Geometry: final body of the model. Coordinates: model frame, mm. Face numbers are marked on the shaded views. A direction names the side the tool comes from. Give positions to 0.01 mm unless a question says otherwise; leave off trailing zeros. Loops run counter-clockwise (first coordinate to the right, second up) from the corner with the lowest first, then second, coordinate; pieces in that order, holes last.
from build123d import *

# Parameters (mm, degrees)
CYLINDER028_R     = 1.25
CYLINDER028_DEPTH = 10
BOX030_W          = 34
BOX030_H          = 2.75
BOX030_DEPTH      = 2
CYLINDER025_W     = 4
CYLINDER025_H     = 26
CYLINDER025_ANGLE = 180


with BuildPart() as b_no002:
    # Cylinder028 → Cylinder028 (new body)
    with BuildSketch(Plane(origin=(11, 29, 4), x_dir=(1, 0, 0), z_dir=(0, 0, 1))):
        Circle(CYLINDER028_R)
    extrude(amount=CYLINDER028_DEPTH)


with BuildPart() as n016:
    # Box030 → Box030 (new body)
    with BuildSketch(Plane(origin=(-3, 25.25, 10), x_dir=(1, 0, 0), z_dir=(0, 0, 1))):
        with Locations((17, 1.375)):
            Rectangle(BOX030_W, BOX030_H)
    extrude(amount=BOX030_DEPTH)


with BuildPart() as obj1:
    # Cylinder025 → Cylinder025 (revolve)
    with BuildSketch(Plane(origin=(11, 28, -14), x_dir=(1, 0, 0), z_dir=(0, -1, 0))):
        with Locations((2, 13)):
            Rectangle(CYLINDER025_W, CYLINDER025_H)
    revolve(axis=Axis((11, 28, -14), (0, 0, 1)), revolution_arc=CYLINDER025_ANGLE)

    # Fusion005: union N016
    add(n016.part)

    # Cut011: cut B_NO002
    add(b_no002.part, mode=Mode.SUBTRACT)


with BuildPart() as obj1_1:
    # Cut011 placement: moved
    add(obj1.part.moved(Location((13, 15, 0))))


solid = obj1_1.part
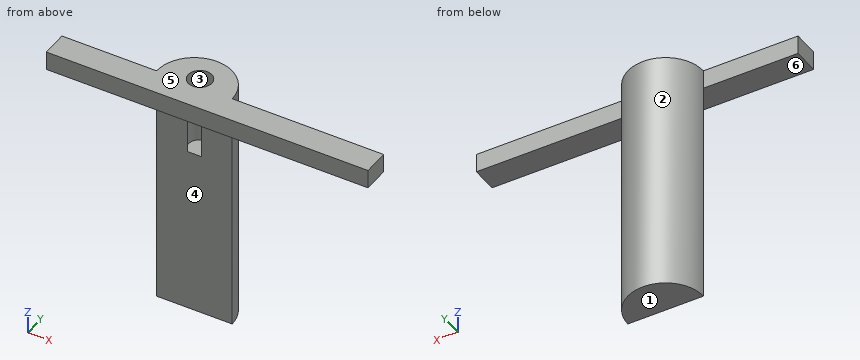
Item 1: Section query A-A on x = 24. Return loops of the section in (y, z).
Values follow:
outline: (40.25, 10) - (42.75, 10) - (42.75, 12) - (40.25, 12) - close; (43, -14) - (47, -14) - (47, 12) - (45.25, 12) - (45.25, 4) - (43, 4) - close
Item 2: Section query D-D on x = 32. Return loops of the section in (y, z).
Values follow:
outline: (40.25, 10) - (43, 10) - (43, 12) - (40.25, 12) - close
Item 3: Pin query (flat end, axial travel): pin 1 (1.1 mm diameter, centred on x = 24, y = 44.5, fed in from +Z); pin 2 (12 mm diameter, centred on x = 19, z = -8.5, fed in from -Y); pin 3 (1.6 mm diameter, centred on x = 17.5, z = 11, fed in from +Y). Return the tip coordinate at first contact, or that it passes through.
Values follow:
pin 1: stops at z = 4
pin 2: stops at y = 43
pin 3: stops at y = 43
Item 4: Section query C-C on z = -3.75. Return loops of the section in (x, y).
Values follow:
outline: (20, 43) - (28, 43) arc R4 ccw to start
Item 5: Ray query, probe 1 along Z at (x, y) = (31, 41.5); probe 2 along X at (y, z) = (45, 7.25); probe 3 along Y at (x, z) = (33, 10.25). Return the intervals inside material, ascending.
Values follow:
probe 1: z = 10 to 12
probe 2: x = 20.54 to 23.25, 24.75 to 27.46
probe 3: y = 40.25 to 43
Item 6: Draft query along Y for the marked faces 1, 2, 3 and 4. Return one class per face: +Y half, -Y half, draft (parallel to the pull), parting line (faces both ways), or undercut.
Values follow:
face 1: draft
face 2: +Y half
face 3: undercut
face 4: -Y half
Item 7: Section query B-B on y = 41.5. Return loops of the section in (x, z), plus the area to 3 significant figures.
Values follow:
outline: (10, 10) - (44, 10) - (44, 12) - (10, 12) - close
area: 68.0 mm2
Item 8: Set-up query: the marked faces 5 and 6. Return all of +Z, -Z, +X, -X, +Y, -Y with unobstructed straight access to the full face (end or side cutting, diameter ignored); none if empty.
Values follow:
face 5: +Z, +X, -X, +Y, -Y
face 6: -Z, +X, -X, -Y
